Drawing for the job (mm, zero at the part's lowest x, y, z). A direction names the side the tool comes from. Give positions to 0.01 mm unless a question says otherwise; leave off trailing zeros. Order: outer loops, then holes, each group sorted by start corner. A loop starts at its lowest first (then second) coordinate and runs counter-clockwise, first axis right, second up. Notation, with made-up numbers: (38.5, 50) - (86.5, 50) arc R19 cw to (86.5, 64) - close; hole circle Ø8 at (-14, -11). An arc over 180 degrees is marked (long way). Use a Markdown table: item, result. Add a question column.
(1) Mould opens along X. For the marked faces 1, 2, 3 and 4 say: +X half, -X half, draft (parallel to the pull), parting line (faces both ways), or undercut.
(2) Flat gauge pins, fed straight in: pin 1 (2 mm diameter, centred on x = 9, z = 5, fed in from -Y); pin 2 (6 mm diameter, centred on x = 3, y = 45, fed in from +Z); pin 3 (1.8 mm diameter, centred on x = 7.5, z = 1.5, fed in from -Y). Where does each tip first touch, or does it go through?
(3) Which spindle directions (+Z, -Z, +X, -X, +Y, -Y) get a long thin tool onto all of the face, cutting with end or side? Do the marked faces 5 and 6. Say none if no direction does.
(4) Slice it at A-A (x = 1.25). Count the separate pieces of the cut face and the enclosed holes in it, then the cut area to 3 significant figures.
(5) Wall check: line 1 (Y direction, x = 2.35, z = 3); line 2 (X direction, y = 5.5, z = 0.5); line 3 (Y direction, x = 10, z = 2). Give the ranges that are in metal, low to high.
(6) Slice it at D-D (y = 16). Write the cut outline in (x, z), then the cut area to 3 significant figures.
(7) Slice it at B-B (y = 5). Write the cut outline in (x, z), then the cut area to 3 significant figures.
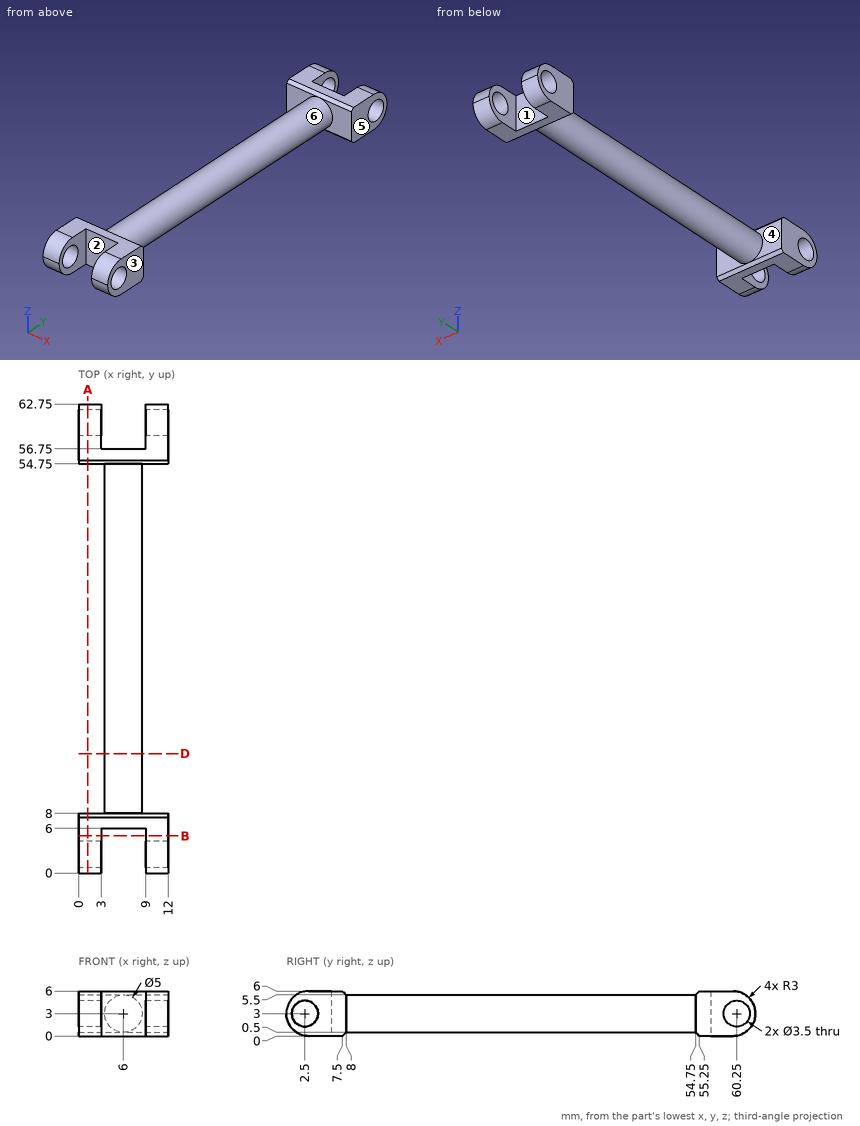
Solution:
| question | item | result |
|---|---|---|
| 1 | face 1 | undercut |
| 1 | face 2 | undercut |
| 1 | face 3 | +X half |
| 1 | face 4 | draft |
| 2 | pin 1 | y = 0.17 |
| 2 | pin 2 | z = 5.5 |
| 2 | pin 3 | y = 6 |
| 3 | face 5 | +Z, -Z, +X, +Y, -Y |
| 3 | face 6 | none |
| 4 | separate pieces | 2 |
| 4 | enclosed holes | 2 |
| 4 | area | 68.5 mm2 |
| 5 | line 1 | 0 to 0.75, 4.25 to 8, 54.75 to 58.5, 62 to 62.75 |
| 5 | line 2 | 0 to 3, 9 to 12 |
| 5 | line 3 | 0.17 to 1.06, 3.94 to 8, 54.75 to 58.81, 61.69 to 62.58 |
| 6 | outline | circle Ø5 at (6, 3) |
| 6 | area | 19.6 mm2 |
| 7 | outline | (0, 0) - (3, 0) - (3, 6) - (0, 6) - close; (9, 0) - (12, 0) - (12, 6) - (9, 6) - close |
| 7 | area | 36.0 mm2 |
